Source: CAD feature listing. Evaluate the final solid. Frame: model axes, mm. Give positions to 0.01 mm unless a question says otherwise; leave off trailing zeros. Order: outer loops, then holes, each group sorted by start corner. A loop starts at its lowest first (then second) coordinate and runs counter-clockwise, first axis right, second up. Notation, with made-up numbers: (48.25, 9.5) - (85.25, 9.5) arc R22 cw to (85.25, 39.5) - close; hole circle Ø9 at (54, 77). An arc over 180 degrees is marked (long way). Answer as CSV lines item,"result".
```python
from build123d import *

# Parameters (mm, degrees)
ESBO_O1_W                = 6
ESBO_O1_H                = 20
RESSALTO_EXTRUS_O1_DEPTH = 6


with BuildPart() as part:
    # Esboço1 → Ressalto-extrusão1 (new body)
    with BuildSketch(Plane.XY):
        Polygon((194, 150), (200, 150), (200, 175), (194, 175), (194, 194), (175, 194), (175, 200), (150, 200), (150, 194), (125, 194), (125, 200), (100, 200), (100, 194), (75, 194), (75, 200), (50, 200), (50, 194), (25, 194), (25, 200), (0, 200), (0, 175), (6, 175), (6, 150), (0, 150), (0, 125), (6, 125), (6, 100), (0, 100), (0, 75), (6, 75), (6, 50), (0, 50), (0, 25), (6, 25), (6, 6), (25, 6), (25, 0), (50, 0), (50, 6), (75, 6), (75, 0), (100, 0), (100, 6), (125, 6), (125, 0), (150, 0), (150, 6), (175, 6), (175, 0), (200, 0), (200, 25), (194, 25), (194, 50), (200, 50), (200, 75), (194, 75), (194, 100), (200, 100), (200, 125), (194, 125), align=None)
        Polygon((100, 76.5), (90, 76.5), (90, 82.5), (100, 82.5), (110, 82.5), (110, 76.5), align=None, mode=Mode.SUBTRACT)
        with Locations((73.5, 100)):
            Rectangle(ESBO_O1_W, ESBO_O1_H, mode=Mode.SUBTRACT)
        Polygon((110, 117.5), (100, 117.5), (90, 117.5), (90, 123.5), (100, 123.5), (110, 123.5), align=None, mode=Mode.SUBTRACT)
        with Locations((126.5, 100)):
            Rectangle(ESBO_O1_W, ESBO_O1_H, mode=Mode.SUBTRACT)
    extrude(amount=RESSALTO_EXTRUS_O1_DEPTH)


solid = part.part
```
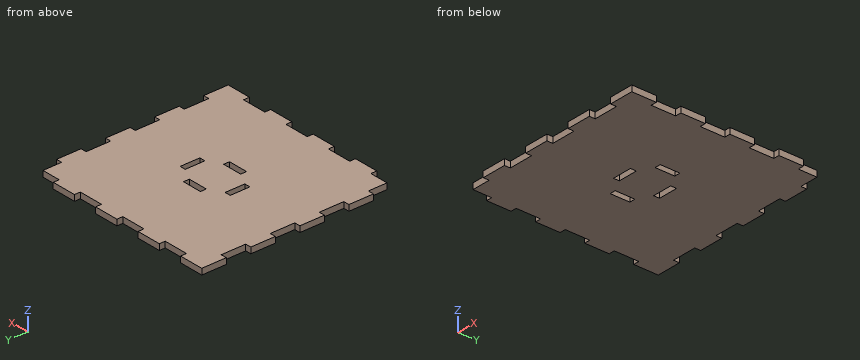
(1) Ray query, line 1 (X direction, y = 90.5, z = 3.95); line 2 (X direction, y = 106, z = 5.1); line 3 (Y direction, x = 103, z = 1.35). Return the intervals inside material, ascending. Write a range as from..to.
Completed:
line 1,"0..70.5, 76.5..123.5, 129.5..194"
line 2,"6..70.5, 76.5..123.5, 129.5..200"
line 3,"6..76.5, 82.5..117.5, 123.5..200"
(2) Contact query for flat-ended pins moving along their axis: pin 1 (3 mm diameter, centred on y = 110, z = 4, fed in from -X); pin 2 (3 mm diameter, centred on x = 42.5, z = 4, fed in from +Y); pin 3 (6 mm diameter, centred on x = 66, y = 82, fed in from -Z); pin 4 (3 mm diameter, centred on y = 3.5, z = 3, fed in from -X). Output: stop coordinate, or through.
Completed:
pin 1,"x = 6"
pin 2,"y = 194"
pin 3,"z = 0"
pin 4,"x = 25"
(3) Cut plane A-A (x = 97). Return loops of the section in (y, z), then the cut area to 3 significant figures.
Completed:
outline,"(0, 0) - (76.5, 0) - (76.5, 6) - (0, 6) - close; (82.5, 0) - (117.5, 0) - (117.5, 6) - (82.5, 6) - close; (123.5, 0) - (194, 0) - (194, 6) - (123.5, 6) - close"
area,"1,090 mm²"
(4) Cut plane D-D (y = 66). Return loops of the section in (x, z), then the cut area to 3 significant figures.
Completed:
outline,"(6, 0) - (200, 0) - (200, 6) - (6, 6) - close"
area,"1,160 mm²"
(5) Cut plane B-B (y = 121). Return loops of the section in (x, z), then the cut area to 3 significant figures.
Completed:
outline,"(6, 0) - (90, 0) - (90, 6) - (6, 6) - close; (110, 0) - (200, 0) - (200, 6) - (110, 6) - close"
area,"1,040 mm²"
(6) Cut plane C-C (z = 4.35). Give the number of separate pieces and of enclosed holes in the cut face, then the cut area to 3 significant figures.
Completed:
separate pieces,"1"
enclosed holes,"4"
area,"37,200 mm²"
